Work out the finished part from the listing and answer in its coordinate system (mm). Face numbers are marked on the shaded views. A direction names the side the tool comes from. Coordinates: 2 decimals unless noted, no trailing zeros. Order: outer loops, then holes, each group sorted by start corner. A loop starts at its lowest first (then second) coordinate and runs counter-clockwise, first axis right, second up.
```python
from build123d import *

# Parameters (mm, degrees)
SKETCH1_R           = 4
BOSS_EXTRUDE1_DEPTH = 10
SKETCH2_R           = 2.475
BOSS_EXTRUDE2_DEPTH = 5
SKETCH3_W           = 1.5
SKETCH3_H           = 5.4
SKETCH3_W_2         = 5.4
SKETCH3_H_2         = 1.5
BOSS_EXTRUDE3_DEPTH = 5
FILLET3_R           = 0.5


with BuildPart() as part:
    # Sketch1 → Boss-Extrude1 (new body)
    with BuildSketch(Plane(origin=(0, 0, 0), x_dir=(1, 0, 0), z_dir=(0, 1, 0))):
        Circle(SKETCH1_R)
    extrude(amount=-BOSS_EXTRUDE1_DEPTH)

    # Sketch2 → Boss-Extrude2 (add)
    with BuildSketch(Plane(origin=(0, 0, 0), x_dir=(1, 0, 0), z_dir=(0, 1, 0))):
        Circle(SKETCH2_R)
    extrude(amount=BOSS_EXTRUDE2_DEPTH)

    # Sketch3 → Boss-Extrude3 (add)
    with BuildSketch(Plane.XZ.offset(10)):
        Rectangle(SKETCH3_W, SKETCH3_H)
        Rectangle(SKETCH3_W_2, SKETCH3_H_2)
    extrude(amount=BOSS_EXTRUDE3_DEPTH)

    # Fillet3
    fillet3_edges = [part.edges().sort_by_distance(p)[0] for p in [
        (-2.475, 5, 0),
    ]]
    fillet(fillet3_edges, radius=FILLET3_R)


solid = part.part
```
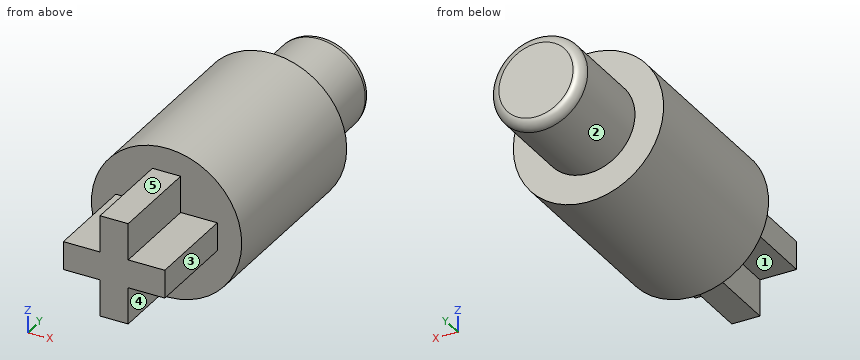
1. Flat-ended cylindrical pins translate along their axes: pin 1 (2 mm diameter, centred on x = -2, y = -13, fed in from +Z); pin 2 (0.6 mm diameter, centred on y = -13, z = -2, fed in from -X); pin 3 (1.2 mm diameter, centred on x = -0.5, y = -13, fed in from +Z). Find the tip coordinate at first contact, or state that the pin passes through.
2. Consider probe 1 along Y at (x, z) = (-2.25, 2.5); probe 2 along Y at (x, z) = (0.5, -2.5); probe 3 along X at (y, z) = (2, 0) (3 decimals). Determine where each line is inside the solid, lowest interval first.
3. The part is cut by section D-D (y = -6.5). Determine the outline of the cut face in (x, z).
4. For the marked faces 1, 2, 3, 4 and 5, determine the directions among +Z, -Z, +X, -X, +Y, -Y from which every point of the face is accessible in a straight line to the end or side of a thin tool.
5. The part is cut by section B-B (x = 0). Determine the outline of the cut face in (y, z) (3 decimals), plus the area to 3 significant figures.
6. The part is cut by section C-C (y = -10.25). Determine the outline of the cut face in (x, z), plus the area to 4 significant figures.
7. The part is cut by section A-A (z = 0). Determine the outline of the cut face in (x, y) (3 decimals).
Worked out:
1. pin 1: stops at z = 0.75
1. pin 2: stops at x = -0.75
1. pin 3: stops at z = 2.7
2. probe 1: y = -10 to 0
2. probe 2: y = -15 to 0
2. probe 3: x = -2.475 to 2.475
3. outline: circle Ø8 at (0, 0)
4. face 1: -Z, -X, -Y
4. face 2: +Y
4. face 3: +Z, -Z, +X, -Y
4. face 4: -Z, +X, -Y
4. face 5: +Z, +X, -X, -Y
5. outline: (-15, -2.7) - (-10, -2.7) - (-10, -4) - (0, -4) - (0, -2.475) - (4.5, -2.475) arc R0.5 ccw to (5, -1.975) - (5, 1.975) arc R0.5 ccw to (4.5, 2.475) - (0, 2.475) - (0, 4) - (-10, 4) - (-10, 2.7) - (-15, 2.7) - close
5. area: 132 mm2
6. outline: (-2.7, -0.75) - (-0.75, -0.75) - (-0.75, -2.7) - (0.75, -2.7) - (0.75, -0.75) - (2.7, -0.75) - (2.7, 0.75) - (0.75, 0.75) - (0.75, 2.7) - (-0.75, 2.7) - (-0.75, 0.75) - (-2.7, 0.75) - close
6. area: 13.95 mm2
7. outline: (-4, -10) - (-2.7, -10) - (-2.7, -15) - (2.7, -15) - (2.7, -10) - (4, -10) - (4, 0) - (2.475, 0) - (2.475, 4.5) arc R0.5 ccw to (1.975, 5) - (-1.975, 5) arc R0.5 ccw to (-2.475, 4.5) - (-2.475, 0) - (-4, 0) - close
